Here's the drawing with two shaded views (mm, measured from the low corner). I have some questions. A direction names the side the tool comes from. Give positions to 0.01 mm unless a question says otherwise; leave off trailing zeros. Order: outer loops, then holes, each group sorted by start corner. A loop starts at its lowest first (then second) coordinate and runs counter-clockwise, first axis right, second up. Notation, with made-up numbers: M 54.5,-35 L 72.5,-35 A10 cw 72.5,-21 Z; hole C 50,-20 d7. An arc over 180 degrees is marked long. Write each question's results on one line, items separated by ' | '.
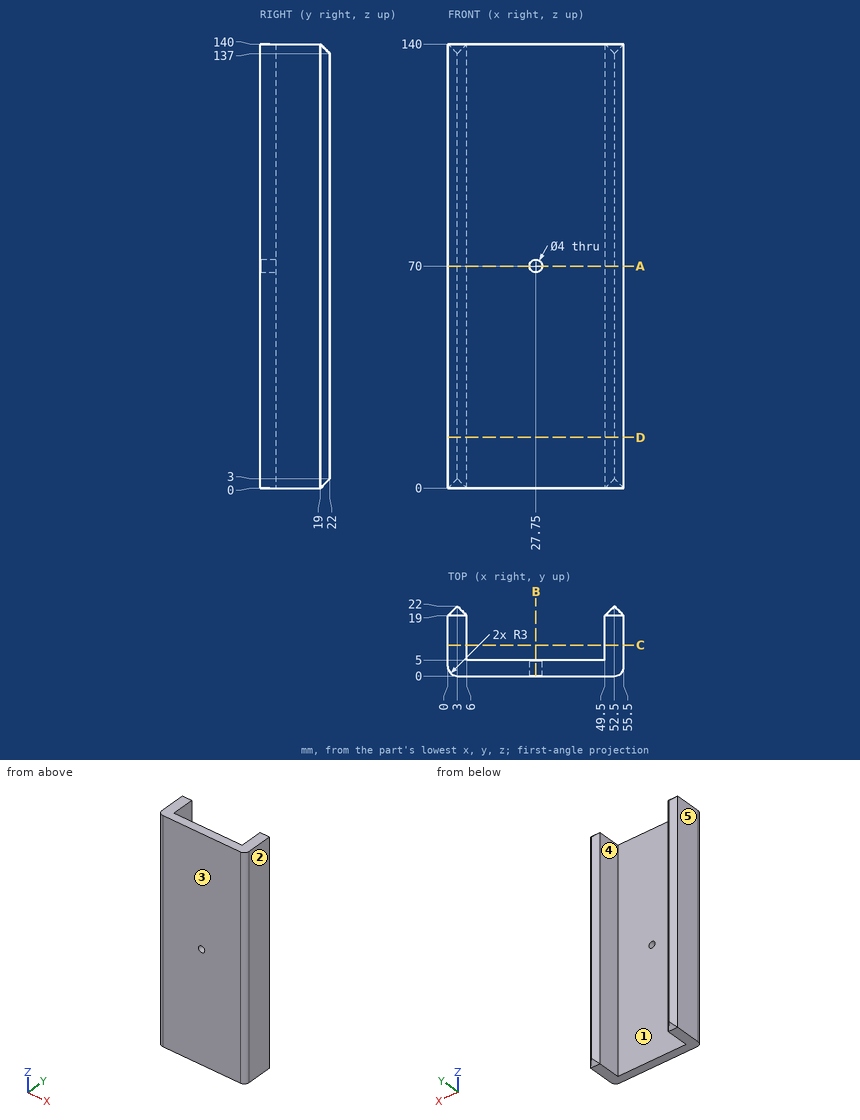
(1) For the marked faces 4 and 5, which set-ups out of +Z, -Z, +X, -X, +Y, -Y let a thin tool reach every point of the face, with its end or its side?
Data:
face 4: +Z, -Z, +Y | face 5: +Z, -Z, -X, +Y, -Y
(2) I need wall thicknesses on L1, parallel to X at y = 3.1, z = 70; L2, parallel to X at y = 18.75, z = 18.5; L3, parallel to Y at x = 8.5, z = 53.5. Which ranges of each line are inside material? Lowest first, please. Write a range as from..to.
Data:
L1: x = 0..25.75, 29.75..55.5 | L2: x = 0..6, 49.5..55.5 | L3: y = 0..5
(3) Imagine slicing it at A-A, the plane z = 70. Write out the boundary of the cut face in (x, y).
Data:
outline: M 0,3 A3 ccw 3,0 L 25.75,0 L 25.75,5 L 6,5 L 6,19 L 3,22 L 0,19 Z; M 29.75,0 L 52.5,0 A3 ccw 55.5,3 L 55.5,19 L 52.5,22 L 49.5,19 L 49.5,5 L 29.75,5 Z
(4) Imagine slicing it at D-D, the plane z = 16. Write out the boundary of the cut face in (x, y), plus the area to 3 significant figures.
Data:
outline: M 0,3 A3 ccw 3,0 L 52.5,0 A3 ccw 55.5,3 L 55.5,19 L 52.5,22 L 49.5,19 L 49.5,5 L 6,5 L 6,19 L 3,22 L 0,19 Z | area: 460 mm2
(5) Will these pins go through, and if not, where does the flat tip stop? P1, Ø12, axis at x = 47.5, y = 5, coming from the -Z side; P2, Ø5, axis at x = 42, z = 34.5, coming from the +Y side.
Data:
P1: stops at z = 0 | P2: stops at y = 5
(6) Imagine slicing it at C-C, the plane y = 9.75. Write out the boundary of the cut face in (x, z).
Data:
outline: M 0,0 L 6,0 L 6,140 L 0,140 Z; M 49.5,0 L 55.5,0 L 55.5,140 L 49.5,140 Z
(7) Imagine slicing it at B-B, the plane x = 27.75. Write out the boundary of the cut face in (y, z).
Data:
outline: M 0,0 L 5,0 L 5,68 L 0,68 Z; M 0,72 L 5,72 L 5,140 L 0,140 Z
(8) We'd pull the mould along X, two halves only. Please class the marked faces 1, 2 and 3: +X half, -X half, draft (parallel to the pull), parting line (faces both ways), or undercut.
Data:
face 1: undercut | face 2: +X half | face 3: draft
